Part model, mm, in its own coordinate system. Give positions to 0.01 mm unless a question says otherwise; leave off trailing zeros. Order: outer loops, then holes, each group sorted by start corner. A loop starts at its lowest first (then second) coordinate and runs counter-clockwise, first axis right, second up. Notation, with made-up numbers: (-22, -10.5) -> (1, -10.5) arc R21 cw to (1, 21.5) -> close; hole circle Ø3 at (-20, -10). An arc over 180 degrees is marked (long way). Write item = value, one per line. Start each with the question number.
(1) Saw through at B-B, the plane y = 27. List the corners of the cut face in (x, z), then the cut area to 3 significant figures.
(2) Saw through at C-C, the plane x = 16. List the corners of the cut face in (y, z).
(3) Saw through at A-A, the plane z = 821. List the corners of the cut face in (x, y).
(4) Probe line 1 along Y through (x, z) = (21.5, 986); line 2 along Y through (x, z) = (3, 255). List the from-to ranges inside material, lowest first. Write a range as from..to.
(5) Flat gauge pins, fed straight in: pin 1 (13 mm diameter, centred on x = 23, z = 283.5, fed in from +Y); pin 2 (8 mm diameter, centred on x = 10, z = 408.5, fed in from +Y); pin 3 (4 mm diameter, centred on y = 24.5, z = 233, fed in from -X); pin 4 (8 mm diameter, centred on y = 31, z = 439.5, fed in from +X). Where does each tip first touch, or does it go through?
Autodesk Inventor part; units mm, degrees
ref_plane "Start plane" through (0, 0, 0) normal (0, 0, 1) x (1, 0, 0)
ref_plane "End plane" through (0, 0, 1066.8) normal (0, 0, 1) x (1, 0, 0)
ref_plane "Work Plane4" through (0, 19.05, 1066.8) normal (0.7071, 0, 0.7071) x (0.7071, 0, -0.7071)
ref_plane "Start plane" through (0, 0, 0) normal (0, 0, 1) x (1, 0, 0)
ref_plane "End plane" through (0, 0, 1066.8) normal (0, 0, 1) x (1, 0, 0)
sketch "Sketch" plane through (0, 0, 0) normal (0, 0, 1) x (1, 0, 0)
  line L0 (38.1, 0) -> (0, 0)
  line L1 (0, 0) -> (0, 38.1)
  line L2 (0, 38.1) -> (2.4765, 38.1)
  line L3 (4.7625, 35.814) -> (4.7625, 9.5885)
  line L4 (9.5885, 4.7625) -> (35.814, 4.7625)
  line L5 (38.1, 2.4765) -> (38.1, 0)
  line L6 (0, -11.0414) -> (0, 31.5385) construction
  line L7 (-11.0414, 0) -> (31.5385, 0) construction
  arc A0 (4.7625, 9.5885) -> (9.5885, 4.7625) centre (9.5885, 9.5885) ccw
  arc A1 (4.7625, 35.814) -> (2.4765, 38.1) centre (2.4765, 35.814) ccw
  arc A2 (38.1, 2.4765) -> (35.814, 4.7625) centre (35.814, 2.4765) ccw
  line L8 (0, 48.4964) -> (0, -20.9644) construction
  line L9 (-20.9644, 0) -> (48.4964, 0) construction
  point P0 (4.7625, 38.1)
  point P1 (4.7625, 4.7625)
  point P2 (38.1, 4.7625)
  dimension "d0" = 38.1
  dimension "d1" = 38.1
  dimension "d2" = 4.7625
  dimension "d3" = 4.7625
  dimension "d10" = 0
  dimension "d11" = 0
  dimension "d14" = 4.826
  dimension "d15" = 2.286
extrude "Body" add sketch "Sketch" along normal up to surface (1066.8 mm away) from surface at 0
sketch "Sketch3" plane through (0, 0, 0) normal (0, 0, 1) x (1, 0, 0)
  line L0 (0, 0) -> (10, 0)
ref_plane "Work Plane3" through (0, 0, 0) normal (0, -1, 0) x (1, 0, 0)
sketch "Sketch4" plane through (0, 0, 0) normal (0, -1, 0) x (1, 0, 0)
  line L0 (-2, 0) -> (12, 0)
  line L1 (-2, 1066.8) -> (12, 1066.8)
  dimension "d17" = 1066.8
ref_plane "Work Plane4" through (0, 19.05, 1066.8) normal (0.7071, 0, 0.7071) x (0.7071, 0, -0.7071)
split "Split1" plane through (0, 19.05, 1066.8) removes the side toward (0.7071, 0, 0.7071)
ref_plane "Work Plane5" through (0, 19.05, 0) normal (0.7071, 0, -0.7071) x (-0.7071, 0, -0.7071)
split "Split2" plane through (0, 19.05, 0) removes the side toward (0.7071, 0, -0.7071)
equation "\"d0\" = G_H"
equation "\"d1\" = G_H"
equation "\"d2\" = G_T"
equation "\"d3\" = G_T"
equation "\"d14\" = G_IR"
equation "\"d15\" = G_ER"
equation "\"d4\" = G_L"
equation "\"G_H\" = 38.1"
equation "\"G_T\" = 4.7625"
equation "\"G_ER\" = 2.286"
equation "\"G_IR\" = 4.826"
equation "\"G_L\" = d17"
equation "\"ex\" = 0"
equation "\"G_OFFSET_START\" = 0"
equation "\"G_OFFSET_END\" = 0"
equation "\"d13\" = G_OFFSET_END + B_L"
equation "\"B_L\" = 1066.8"
properties part number "AISC - L 1.5 x 1.5 x 3/16 - 42" material "Aluminum 6061-AHC"
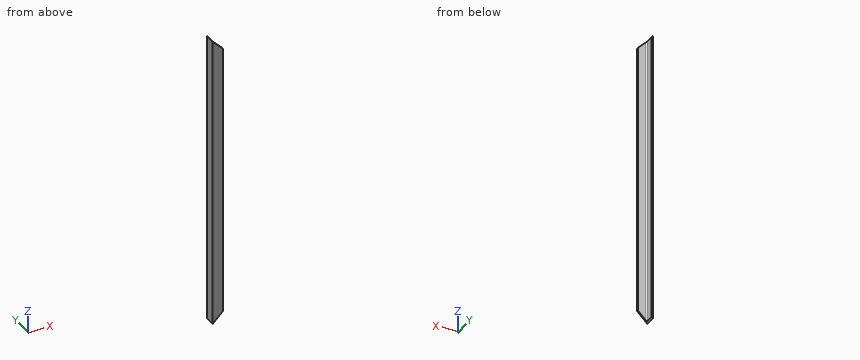
Results list:
q1.outline = (0, 0) -> (4.76, 4.76) -> (4.76, 1062.04) -> (0, 1066.8) -> close
q1.area = 5,060 mm^2
q2.outline = (0, 16) -> (4.76, 16) -> (4.76, 1050.8) -> (0, 1050.8) -> close
q3.outline = (0, 0) -> (38.1, 0) -> (38.1, 2.48) arc R2.29 ccw to (35.81, 4.76) -> (9.59, 4.76) arc R4.83 cw to (4.76, 9.59) -> (4.76, 35.81) arc R2.29 ccw to (2.48, 38.1) -> (0, 38.1) -> close
q4.line_1 = 0..4.76
q4.line_2 = 0..38.04
q5.pin_1 = 4.76
q5.pin_2 = 6.36
q5.pin_3 = 0
q5.pin_4 = 4.76
